Here's how the part is built. I have some questions about the finished solid (model axes, mm). Give positions to 0.01 mm unless a question says otherwise; leave off trailing zeros. Loops run counter-clockwise (first coordinate to the right, second up) from the corner with the lowest first, then second, coordinate; pieces in that order, holes last. Notation, with made-up numbers: (-22.5, 55.5) -> (10.5, 55.5) arc R25 cw to (10.5, 89.5) -> close; hole circle Ø9 at (0, -3.5). An arc over 180 degrees is marked (long way). Answer in a Markdown table with one row per item. Add a question column.
Item 1: For P1, Ø4.5, axis at x = 185, z = -15, coming from the +Y side; P2, Ø8, axis at x = 15, z = -15, coming from the -Y side, each with a flat end and sliding along its axis, tell me the tip position at first contact or that it passes through.
Item 2: If I drill on line 1 (Z direction, x = 185, y = 3); line 2 (X direction, y = 2.6, z = -185); line 3 (Z direction, x = 116, y = 3.6), over which ranges is the centre line in solid material (lowest first)?
Item 3: If we section it at C-C (y = 1.8): Write out the boundary of the cut face in (x, z), then the cut area to 3 significant figures.
Item 4: If we section it at D-D (x = 185): Write out the boundary of the cut face in (y, z), then the cut area to 3 significant figures.
Item 5: If we section it at A-A (z = -185): Write out the boundary of the cut face in (x, y), then the cut area to 3 significant figures.
Item 6: If we section it at B-B (x = 111): Write out the boundary of the cut face in (y, z).
```python
from build123d import *

# Parameters (mm, degrees)
CROQUIS1_W              = 200
CROQUIS1_H              = 200
CROQUIS1_R              = 2.5
SALIENTE_EXTRUIR1_DEPTH = 4
CROQUIS2_W              = 100
CROQUIS2_H              = 100
CORTAR_EXTRUIR1_DEPTH   = 4


with BuildPart() as part:
    # Croquis1 → Saliente-Extruir1 (new body)
    with BuildSketch(Plane(origin=(0, 0, 0), x_dir=(1, 0, 0), z_dir=(0, 1, 0))):
        with Locations((100, 100)):
            Rectangle(CROQUIS1_W, CROQUIS1_H)
        with Locations(Location((15, 185, 0), (0, 0, 270))):
            Circle(CROQUIS1_R, mode=Mode.SUBTRACT)
        with Locations(Location((185, 185, 0), (0, 0, 270))):
            Circle(CROQUIS1_R, mode=Mode.SUBTRACT)
        with Locations(Location((185, 15, 0), (0, 0, 270))):
            Circle(CROQUIS1_R, mode=Mode.SUBTRACT)
        with Locations(Location((15, 15, 0), (0, 0, 270))):
            Circle(CROQUIS1_R, mode=Mode.SUBTRACT)
    extrude(amount=SALIENTE_EXTRUIR1_DEPTH)

    # Croquis2 → Cortar-Extruir1 (cut)
    with BuildSketch(Plane(origin=(0, 4, 0), x_dir=(1, 0, 0), z_dir=(0, 1, 0))):
        with Locations((100, 100)):
            Rectangle(CROQUIS2_W, CROQUIS2_H)
    extrude(amount=-CORTAR_EXTRUIR1_DEPTH, mode=Mode.SUBTRACT)


solid = part.part
```
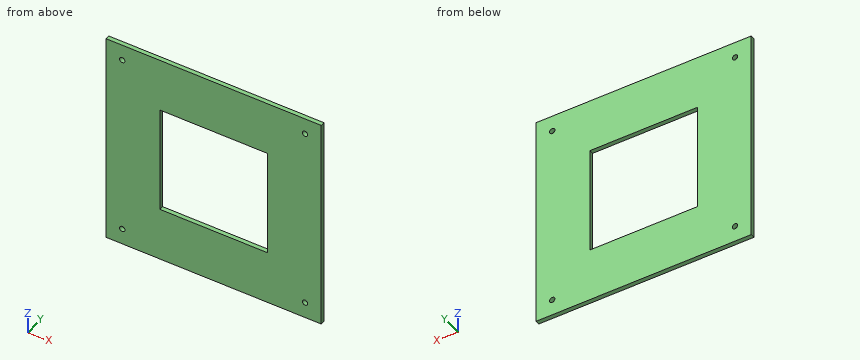
Recorded:
| question | item | result |
|---|---|---|
| 1 | P1 | passes through |
| 1 | P2 | stops at y = 0 |
| 2 | line 1 | z = -200 to -187.5, -182.5 to -17.5, -12.5 to 0 |
| 2 | line 2 | x = 0 to 12.5, 17.5 to 182.5, 187.5 to 200 |
| 2 | line 3 | z = -200 to -150, -50 to 0 |
| 3 | outline | (0, -200) -> (200, -200) -> (200, 0) -> (0, 0) -> close; hole circle Ø5 at (15, -185); hole circle Ø5 at (15, -15); hole (50, -150) -> (150, -150) -> (150, -50) -> (50, -50) -> close; hole circle Ø5 at (185, -185); hole circle Ø5 at (185, -15) |
| 3 | area | 29,900 mm^2 |
| 4 | outline | (0, -200) -> (4, -200) -> (4, -187.5) -> (0, -187.5) -> close; (0, -182.5) -> (4, -182.5) -> (4, -17.5) -> (0, -17.5) -> close; (0, -12.5) -> (4, -12.5) -> (4, 0) -> (0, 0) -> close |
| 4 | area | 760 mm^2 |
| 5 | outline | (0, 0) -> (12.5, 0) -> (12.5, 4) -> (0, 4) -> close; (17.5, 0) -> (182.5, 0) -> (182.5, 4) -> (17.5, 4) -> close; (187.5, 0) -> (200, 0) -> (200, 4) -> (187.5, 4) -> close |
| 5 | area | 760 mm^2 |
| 6 | outline | (0, -200) -> (4, -200) -> (4, -150) -> (0, -150) -> close; (0, -50) -> (4, -50) -> (4, 0) -> (0, 0) -> close |
